Work out the finished part from the listing and answer in its coordinate system (mm). Face numbers are marked on the shaded views. A direction names the side the tool comes from. Coordinates: 2 decimals unless noted, no trailing zeros. Order: outer loops, then holes, each group sorted by start corner. A loop starts at its lowest first (then second) coordinate and runs counter-clockwise, first axis right, second up. Notation, with made-up numbers: (11, 82) -> (63, 82) arc R25 ccw to (63, 110) -> close; hole circle Ø1 at (22, 82). An arc over 180 degrees is marked (long way). Write item = value, one per line. Start each with the question number.
Q1. The part is cut by section D-D, the plane x = 24.5. Determine the outline of the cut face in (y, z), plus the area to 3 significant figures.
Q2. Straight lines are drawn through the part: L1, parallel to Z at x = 32.5, y = 45.5; L2, parallel to Y at x = 6, z = -7; L3, parallel to Y at x = 21.5, z = -6.75. For each, find the intervals that lie inside material, in ascending order. Write a range as from..to.
Q3. The part is cut by section C-C, the plane x = -21.21. Determine the outline of the cut face in (y, z).
Q4. For a pull along Y with two mould halves and no side action, classify the marked faces 4, 5, 6 and 7 as +Y half, -Y half, draft (parallel to the pull), parting line (faces both ways), or undercut.
Q5. The part is cut by section A-A, the plane x = -8.5. Determine the outline of the cut face in (y, z).
Q6. The part is cut by section B-B, the plane z = -5. Determine the outline of the cut face in (x, y) (1 decimal), plus the area to 3 significant figures.
Q7. Which of the six approach directions +Z, -Z, +X, -X, +Y, -Y give full straight-line access (tool end or side, diameter ignored) to the marked faces 1, 2 and 3?
Q8. Flat-ended cylindrical pins translate along their axes: pin 1 (2 mm diameter, centred on y = 60.5, z = -2.5, fed in from -X); pin 2 (6 mm diameter, centred on y = 43, z = -17.5, fed in from -X); pin 3 (5 mm diameter, centred on x = 16.5, z = -7, fed in from +Y); pin 4 (3 mm diameter, centred on y = 42, z = -3, fed in from -X). Find the tip coordinate at first contact, or state that the pin passes through.
Solid Edge part; units mm, degrees
sketch "Sketch1" plane through (0, 0, 0) normal (0, 0, 1) x (1, 0, 0)
  line L0 (20.754, 21.3618) -> (6.6119, 7.2197)
  line L1 (6.6119, 7.2197) -> (-0.4592, 0.1486)
  line L2 (-0.4592, 0.1486) -> (-52.4074, 52.0969)
  line L3 (-52.4074, 52.0969) -> (-42.3232, 56.1548)
  line L4 (-0.8289, 14.6605) -> (-42.3232, 56.1548)
  line L5 (-0.8289, 14.6605) -> (27.4554, 42.9448)
  line L6 (27.4554, 42.9448) -> (-14.0397, 84.4398)
  line L7 (-14.0397, 84.4398) -> (-9.9823, 94.5245)
  line L8 (41.9672, 42.575) -> (-9.9823, 94.5245)
  line L9 (34.8962, 35.5039) -> (41.9672, 42.575)
  line L10 (20.754, 21.3618) -> (34.8962, 35.5039)
  circle A0 centre (6.6829, 70.6568) radius 2.3
  circle A1 centre (-21.21, 29.0455) radius 2.3
  circle A2 centre (-28.2811, 36.1166) radius 2.3
  circle A3 centre (13.754, 63.5857) radius 2.3
extrude "Protrusion1" add sketch "Sketch1" against normal blind 10
sketch "Sketch2" plane through (0, 0, 0) normal (0, 0, 1) x (1, 0, 0)
  circle A0 centre (6.6829, 70.6568) radius 2.3
extrude "ExtrudedProtrusion_6" add sketch "Sketch2" against normal blind 20
sketch "Sketch3" plane through (0, 0, 0) normal (0, 0, 1) x (1, 0, 0)
  circle A0 centre (13.754, 63.5857) radius 2.3
extrude "ExtrudedProtrusion_7" add sketch "Sketch3" against normal blind 20
sketch "Sketch4" plane through (0, 0, 0) normal (0, 0, 1) x (1, 0, 0)
  circle A0 centre (-28.2811, 36.1166) radius 2.3
extrude "ExtrudedProtrusion_8" add sketch "Sketch4" against normal blind 20
sketch "Sketch5" plane through (0, 0, 0) normal (0, 0, 1) x (1, 0, 0)
  circle A0 centre (-21.21, 29.0455) radius 2.3
extrude "ExtrudedProtrusion_9" add sketch "Sketch5" against normal blind 20
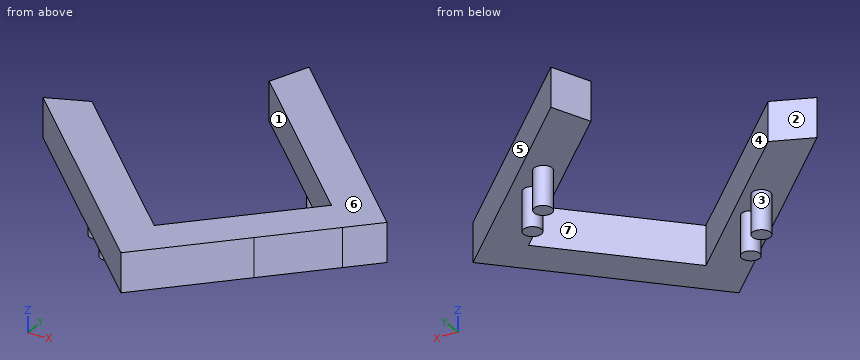
Model answer:
q1.outline = (25.11, -10) -> (39.99, -10) -> (39.99, 0) -> (25.11, 0) -> close; (45.9, -10) -> (60.04, -10) -> (60.04, 0) -> (45.9, 0) -> close
q1.area = 290 mm2
q2.L1 = -10..0
q2.L2 = 6.61..21.49, 64.4..78.54
q2.L3 = 22.11..36.99, 48.9..63.04
q3.outline = (20.9, -10) -> (26.75, -10) -> (26.75, -20) -> (31.35, -20) -> (31.35, -10) -> (35.04, -10) -> (35.04, 0) -> (20.9, 0) -> close
q4.face_4 = undercut
q4.face_5 = +Y half
q4.face_6 = draft
q4.face_7 = undercut
q5.outline = (8.19, -10) -> (22.33, -10) -> (22.33, 0) -> (8.19, 0) -> close; (78.9, -10) -> (93.04, -10) -> (93.04, 0) -> (78.9, 0) -> close
q6.outline = (-52.4, 52.1) -> (-0.5, 0.1) -> (20.8, 21.4) -> (34.9, 35.5) -> (42, 42.6) -> (-10, 94.5) -> (-14, 84.4) -> (27.5, 42.9) -> (-0.8, 14.7) -> (-42.3, 56.2) -> close
q6.area = 1,850 mm2
q7.face_1 = +Z, -Z
q7.face_2 = +Z, -Z, -X, +Y
q7.face_3 = -Z
q8.pin_1 = 8.9
q8.pin_2 = through
q8.pin_3 = 70.54
q8.pin_4 = -43.81
